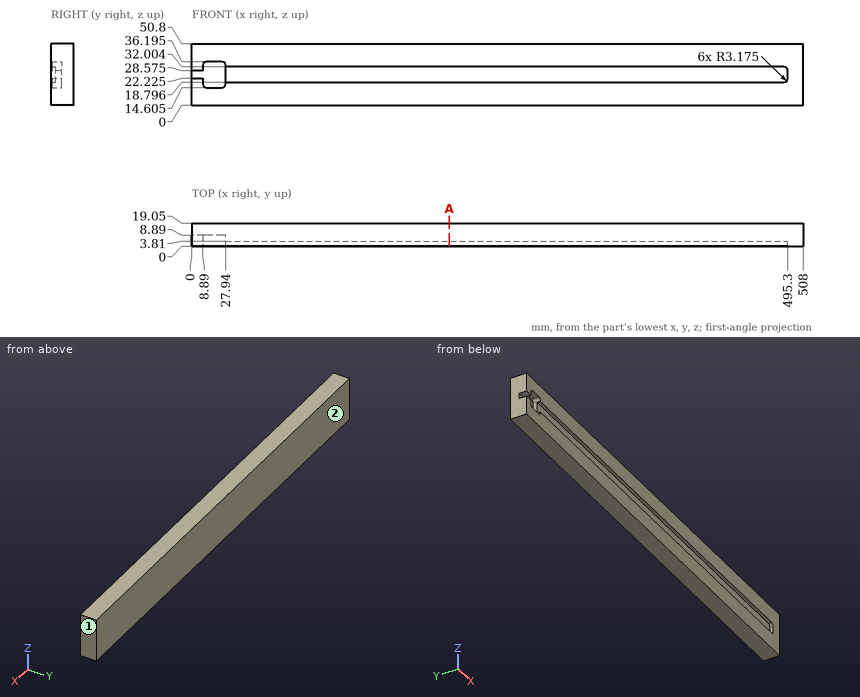
The figure shows three views and two pictorial views of one solid part (mm, origin at its lowest corner). Answer the questions. Coordinates: 2 decimals unless noted, no trailing zeros. Loops run counter-clockwise (first coordinate to the right, second up) from the corner with the lowest first, then second, coordinate; pieces in that order, holes last. Notation, with made-up numbers: (6.5, -26) -> (65.5, -26) arc R9 ccw to (65.5, -13) -> close; hole circle Ø11 at (69.25, -17.5). An arc over 180 degrees is marked (long way). Write item = value, one per line. Start each with the question number.
1) A cutting plane is placed at A-A (x = 214). Give the vertices of the cut face in (y, z), then the cut area to 3 significant figures.
2) Given pin 1 Ø12 at (x, z) = (326, 33) entering from -Y; pin 2 Ø1.9 at (y, z) = (2, 25.5) entering from -X; pin 3 Ø4 at (x, z) = (222, 23.5) entering from -Y, each flat-ended and moving along its own axis, determine where each tip first touches the part or whether it passes through.
3) Straight lines are drawn through the part: line 1 (Z direction, x = 487.5, y = 2.5); line 2 (Y direction, x = 426.5, z = 26.5); line 3 (Y direction, x = 27, z = 21). For each, find the intervals that lie inside material, in ascending order. Write a range as from..to.
4) The mould has two halves that part along Y. Classify the marked faces 1 and 2: released by +Y, released by -Y, zero draft, split by the parting line, or undercut.
Responses:
q1.outline = (0, 0) -> (19.05, 0) -> (19.05, 50.8) -> (0, 50.8) -> (0, 32) -> (3.81, 32) -> (3.81, 18.8) -> (0, 18.8) -> close
q1.area = 917 mm²
q2.pin_1 = 0
q2.pin_2 = 495.3
q2.pin_3 = 3.81
q3.line_1 = 0..18.8, 32..50.8
q3.line_2 = 3.81..19.05
q3.line_3 = 8.89..19.05
q4.face_1 = zero draft
q4.face_2 = released by +Y
